Work out the finished part from the listing and answer in its coordinate system (mm). A direction names the side the tool comes from. Round coordinates to 2 decimals unless told otherwise and drop trailing zeros. Write each loop counter-clockwise with the first axis right and the second up, starting at its lowest first coordinate (ties: lowest second). Pieces come first, ordered by that corner, then holes.
1. Find section A-A (x = 0). Count the separate pieces of the cut face and the enclosed holes in it, and give its area (3 significant figures).
2. Straight lines are drawn through the part: probe 1 along Z at (x, y) = (0, 4.45); probe 2 along Z at (x, y) = (0, 2.85); probe 3 along Z at (x, y) = (0, 3.15). For each, find the intervals that lie inside material, in ascending order.
3. Flat-ended cylindrical pins translate along their axes: pin 1 Ø1.8 at (x, z) = (-9.09, 5.25) entering from +Y; pin 2 Ø5 at (x, z) = (-9.09, -5.25) entering from +Y; pin 3 Ø1.5 at (x, y) = (0, 0.5) entering from -Z; pin 4 Ø3.5 at (x, z) = (0, 10.5) entering from -Y. Find the tip coordinate at first contact, or state that the pin passes through.
4. A tool of negligible diameter and unlimited length cuts with its end or side. For faces 3 (the face through (6, 1.5, 3)), 4 (the face through (-13.712, 2.117, 18.635)), 5 (the face through (-15.346, 2.535, -5.13)), from which of +Z, -Z, +X, -X, +Y, -Y can it reach the whole face along a straight path? Write none if from no direction.
5. Determine the mould class of faces 1 (the face through (27.075, 2.465, 8.899)), 2 (the face through (10, 3, -22)) for opening direction Z: pulls with the +Z half, pulls with the -Z half, needs draft (parallel to the pull), parting line crosses it, or undercut.
6. Find section B-B (z = 10.5). Write down the section's boundary in (x, y), and give its area (3 significant figures).
```python
from build123d import *

# Parameters (mm, degrees)
SKETCH1_R           = 28.5
BOSS_EXTRUDE1_DEPTH = 5
CUT_EXTRUDE1_DEPTH  = 6
CIRPATTERN1_COUNT   = 5
SKETCH3_R           = 14
CUT_EXTRUDE2_DEPTH  = 1.5
SKETCH4_R           = 1.5
SKETCH4_R_2         = 6
CUT_EXTRUDE3_DEPTH  = 4.5
SKETCH5_R           = 1.5
CUT_EXTRUDE4_DEPTH  = 6
CIRPATTERN2_COUNT   = 5
FILLET1_R           = 0.5
SKETCH7_R           = 1
BOSS_EXTRUDE2_DEPTH = 20
CIRPATTERN3_COUNT   = 5


with BuildPart() as part:
    # Sketch1 → Boss-Extrude1 (new body)
    with BuildSketch(Plane(origin=(0, 0, 0), x_dir=(1, 0, 0), z_dir=(0, 1, 0))):
        Circle(SKETCH1_R)
    extrude(amount=BOSS_EXTRUDE1_DEPTH)

    # Sketch2 → Cut-Extrude1 (cut, through all)
    with BuildSketch(Plane(origin=(0, 5, 0), x_dir=(1, 0, 0), z_dir=(0, 1, 0))):
        with BuildLine():
            Line((10, 26.68801229), (10, 17.68801229))
            ThreePointArc((10, 17.68801229), (0, 16.180315356), (-10, 17.68801229))
            Line((-10, 17.68801229), (-10, 26.68801229))
            ThreePointArc((-10, 26.68801229), (0, 28.5), (10, 26.68801229))
        make_face()
    cut_extrude1 = extrude(amount=-CUT_EXTRUDE1_DEPTH, mode=Mode.SUBTRACT)

    # CirPattern1: Cut-Extrude1 ×5 about axis
    cirpattern1_axis = Axis((0, 0, 0), (0, 1, 0))
    for i in range(1, CIRPATTERN1_COUNT):
        add(cut_extrude1.rotate(cirpattern1_axis, i * 360 / CIRPATTERN1_COUNT), mode=Mode.SUBTRACT)

    # Sketch3 → Cut-Extrude2 (cut)
    with BuildSketch(Plane(origin=(0, 5, 0), x_dir=(1, 0, 0), z_dir=(0, 1, 0))):
        Circle(SKETCH3_R)
    cut_extrude2 = extrude(amount=-CUT_EXTRUDE2_DEPTH, mode=Mode.SUBTRACT)

    # Mirror1: Cut-Extrude2 across plane
    add(cut_extrude2.mirror(Plane.ZX.offset(2.5)), mode=Mode.SUBTRACT)

    # Sketch4 → Cut-Extrude3 (cut, through all)
    with BuildSketch(Plane(origin=(0, 3.5, 0), x_dir=(1, 0, 0), z_dir=(0, 1, 0))):
        with Locations((0, 10.5)):
            Circle(SKETCH4_R)
        with Locations((9.09326674, 5.25)):
            Circle(SKETCH4_R)
        with Locations((9.09326674, -5.25)):
            Circle(SKETCH4_R)
        with Locations((0, -10.5)):
            Circle(SKETCH4_R)
        with Locations((-9.09326674, -5.25)):
            Circle(SKETCH4_R)
        with Locations((-9.09326674, 5.25)):
            Circle(SKETCH4_R)
        Circle(SKETCH4_R_2)
    extrude(amount=-CUT_EXTRUDE3_DEPTH, mode=Mode.SUBTRACT)

    # Sketch5 → Cut-Extrude4 (cut, through all)
    with BuildSketch(Plane(origin=(0, 5, 0), x_dir=(1, 0, 0), z_dir=(0, 1, 0))):
        with Locations((0, -24)):
            Circle(SKETCH5_R)
    cut_extrude4 = extrude(amount=-CUT_EXTRUDE4_DEPTH, mode=Mode.SUBTRACT)

    # CirPattern2: Cut-Extrude4 ×5 about axis
    cirpattern2_axis = Axis((0, 0, 0), (0, 1, 0))
    for i in range(1, CIRPATTERN2_COUNT):
        add(cut_extrude4.rotate(cirpattern2_axis, i * 360 / CIRPATTERN2_COUNT), mode=Mode.SUBTRACT)

    # Fillet1
    fillet1_edges = [part.edges().sort_by_distance(p)[0] for p in [
        (-10, 2.5, -26.68801229),
        (10, 2.5, -26.68801229),
        (10, 2.5, -17.68801229),
        (-10, 2.5, -17.68801229),
        (22.291638052, 2.5, -17.757614507),
        (28.471977939, 2.5, 1.263515819),
        (19.912469293, 2.5, 4.044668769),
        (23.776989981, 2.5, 15.713202966),
        (7.596650093, 2.5, 27.468908012),
        (2.306582823, 2.5, 20.187755062),
        (18.48692271, 2.5, 8.432050017),
        (-7.596650093, 2.5, 27.468908012),
        (-23.776989981, 2.5, 15.713202966),
        (-18.48692271, 2.5, 8.432050017),
        (-2.306582823, 2.5, 20.187755062),
        (-28.471977939, 2.5, 1.263515819),
        (-22.291638052, 2.5, -17.757614507),
        (-13.732129405, 2.5, -14.976461557),
        (-19.912469293, 2.5, 4.044668769),
    ]]
    fillet(fillet1_edges, radius=FILLET1_R)

    # Sketch7 → Boss-Extrude2 (add)
    with BuildSketch(Plane(origin=(-8.090169944, 0, -5.877852523), x_dir=(0.587785252, 0, -0.809016994), z_dir=(0.809016994, 0, 0.587785252))):
        with Locations((-24.059120617, 2.5)):
            Circle(SKETCH7_R)
    boss_extrude2 = extrude(amount=BOSS_EXTRUDE2_DEPTH)

    # CirPattern3: Boss-Extrude2 ×5 about axis
    cirpattern3_axis = Axis((0, 3.5, 0), (0, 1, 0))
    for i in range(1, CIRPATTERN3_COUNT):
        add(boss_extrude2.rotate(cirpattern3_axis, i * 360 / CIRPATTERN3_COUNT))


solid = part.part
```
Worked answers:
1. separate pieces: 6
1. enclosed holes: 0
1. area: 91.5 mm2
2. probe 1: z = -16.18 to -14, 14 to 22.5, 25.5 to 28.5
2. probe 2: z = -25 to -23.12, -16.18 to -12, -9 to -6, 6 to 9, 12 to 22.5, 25.5 to 28.5
2. probe 3: z = -24.82 to -23.3, -16.18 to -12, -9 to -6, 6 to 9, 12 to 22.5, 25.5 to 28.5
3. pin 1: passes through
3. pin 2: stops at y = 3.5
3. pin 3: stops at z = -16.19
3. pin 4: stops at y = 1.5
4. face 3: -Y
4. face 4: none
4. face 5: +Y, -Y
5. face 1: pulls with the +Z half
5. face 2: undercut
6. outline: (-26.5, 0) - (-19.99, 0) - (-19.99, 5) - (-26.5, 5) - close; (-13.68, 0) - (-9.26, 0) - (-9.26, 1.5) - (-1.5, 1.5) - (-1.5, 3.5) - (-9.26, 3.5) - (-9.26, 5) - (-13.68, 5) - close; (1.5, 1.5) - (9.26, 1.5) - (9.26, 0) - (13.68, 0) - (13.68, 5) - (9.26, 5) - (9.26, 3.5) - (1.5, 3.5) - close; (19.99, 0) - (26.5, 0) - (26.5, 5) - (19.99, 5) - close
6. area: 140 mm2
